The figure shows three views and two pictorial views of one solid part (mm, origin at its lowest corner). Answer the questions. A direction names the side the tool comes from. Coordinates: 2 decimals unless noted, no trailing zeros. Write each loop counter-clockwise with the first axis right and the second up, starting at its lowest first coordinate (ties: lowest second). Pieces come first, ordered by that corner, then holes. Notation, with made-up numbers: (21, -20.5) - (43, -20.5) arc R24 ccw to (43, -7.5) - close; hole circle Ø3 at (8.25, 19.25). An arc over 180 degrees is marked (long way). Use a Markdown table: item, result. Add a question column.
(1) For a pull along Z with two mould halves and no side action, classify the marked faces 1, 2 and 3 as released by +Z, released by -Z, zero draft, split by the parting line, or undercut.
(2) Given pin 1 Ø20 at (y, z) = (66, 21) entering from +X; pin 2 Ø12.5 at (y, z) = (71.5, 34.5) entering from -X; pin 3 Ø21.5 at (x, z) = (53.5, 32) entering from +Y, each flat-ended and moving along its own axis, determine where each tip first touches the part or whether it passes through.
(3) The part is cut by section A-A, the plane x = 30. Give the vertices of the cut face in (y, z), then the cut area to 3 significant figures.
(4) The part is cut by section B-B, the plane y = 14. Give the vertices of the cut face in (x, z) (1 decimal), then the cut area to 3 significant figures.
(5) Find the intervals of material crossed by line 1 (Z direction, x = 30, y = 30); line 2 (X direction, y = 73.5, z = 5); line 3 (Y direction, x = 10, z = 45.5), in increasing order. Write a range as from..to.
(6) The part is cut by section C-C, the plane z = 30. Give the vertices of the cut face in (x, y), then the cut area to 3 significant figures.
(7) A tool of negligible diameter and unlimited length cuts with its end or side. For the marked faces 4, 5 and 6, from which of +Z, -Z, +X, -X, +Y, -Y can it reach the whole face along a straight path? Write none if from no direction.
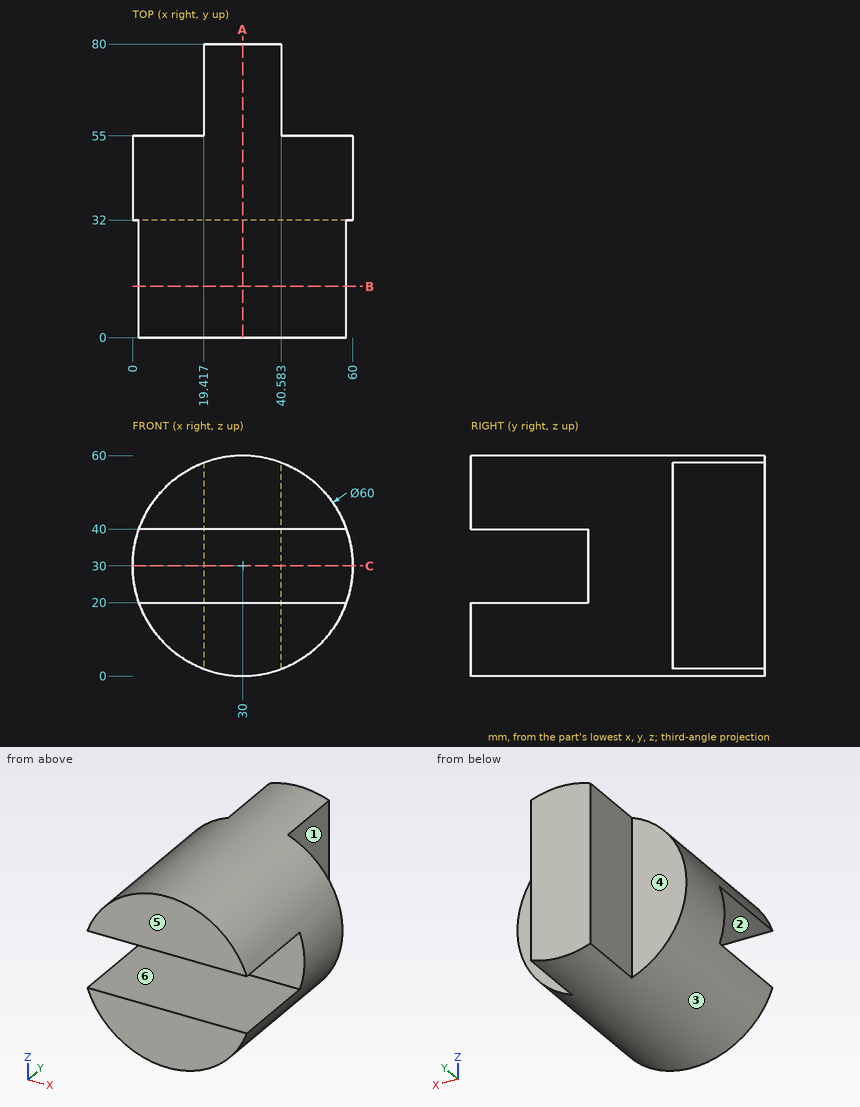
Model answer:
| question | item | result |
|---|---|---|
| 1 | face 1 | zero draft |
| 1 | face 2 | undercut |
| 1 | face 3 | split by the parting line |
| 2 | pin 1 | x = 40.58 |
| 2 | pin 2 | x = 19.42 |
| 2 | pin 3 | y = 55 |
| 3 | outline | (0, 0) - (80, 0) - (80, 60) - (0, 60) - (0, 40) - (32, 40) - (32, 20) - (0, 20) - close |
| 3 | area | 4,160 mm^2 |
| 4 | outline | (1.7, 20) arc R30 ccw to (58.3, 20) - close; (1.7, 40) - (58.3, 40) arc R30 ccw to start |
| 4 | area | 1,650 mm^2 |
| 5 | line 1 | 0..20, 40..60 |
| 5 | line 2 | 19.42..40.58 |
| 5 | line 3 | 0..55 |
| 6 | outline | (0, 32) - (60, 32) - (60, 55) - (40.58, 55) - (40.58, 80) - (19.42, 80) - (19.42, 55) - (0, 55) - close |
| 6 | area | 1,910 mm^2 |
| 7 | face 4 | +Z, -Z, -X, +Y |
| 7 | face 5 | +Z, -Z, +X, -X, -Y |
| 7 | face 6 | +X, -X, -Y |
